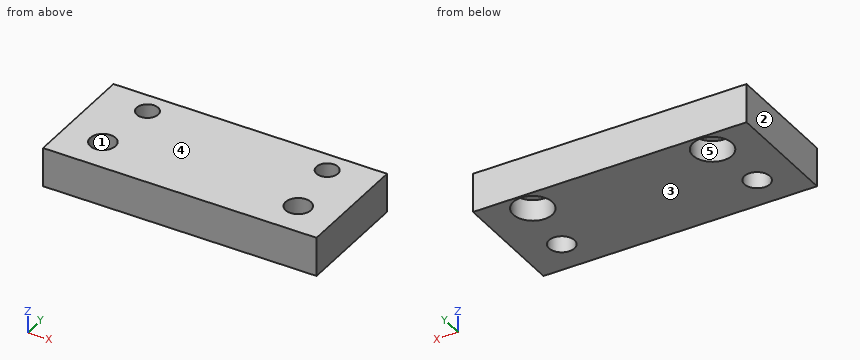
```python
from build123d import *

# Parameters (mm, degrees)
SKETCH1_W           = 70
SKETCH1_H           = 30
SKETCH1_R           = 3.25
SKETCH1_R_2         = 2.75
BOSS_EXTRUDE1_DEPTH = 10
SKETCH3_R           = 5
CUT_EXTRUDE1_DEPTH  = 5.4


with BuildPart() as part:
    # Sketch1 → Boss-Extrude1 (new body)
    with BuildSketch(Plane.XY):
        Rectangle(SKETCH1_W, SKETCH1_H)
        with Locations((-25, -6.150362319)):
            Circle(SKETCH1_R, mode=Mode.SUBTRACT)
        with Locations((25, -6.150362319)):
            Circle(SKETCH1_R, mode=Mode.SUBTRACT)
        with Locations((-23, 9.5)):
            Circle(SKETCH1_R_2, mode=Mode.SUBTRACT)
        with Locations((23, 9.5)):
            Circle(SKETCH1_R_2, mode=Mode.SUBTRACT)
    extrude(amount=BOSS_EXTRUDE1_DEPTH)

    # Sketch3 → Cut-Extrude1 (cut)
    with BuildSketch(Plane(origin=(0, 0, 0), x_dir=(-1, 0, 0), z_dir=(0, 0, -1))):
        with Locations((-23, 9.5)):
            Circle(SKETCH3_R)
        with Locations((23, 9.5)):
            Circle(SKETCH3_R)
    extrude(amount=-CUT_EXTRUDE1_DEPTH, mode=Mode.SUBTRACT)


solid = part.part
```
Verification items for the finished model (mm, model axes). Face numbers are marked on the shaded views. A direction names the side the tool comes from. Coordinates: 2 decimals unless noted, no trailing zeros. Loops run counter-clockwise (first coordinate to the right, second up) from the corner with the lowest first, then second, coordinate; pieces in that order, holes last. Notation, with made-up numbers: (-39, -13) - (-35, -13) arc R22 cw to (-35, -6) - close; hole circle Ø3 at (-34.75, 87). An arc over 180 degrees is marked (long way). Put each result on its own line as item: value.
Item 1: Draft check along X on the marked faces 1, 2 and 3. Enter one of: pulls with the +X half, pulls with the -X half, needs draft (parallel to the pull), parting line crosses it, or undercut.
Conclusion:
face 1: undercut
face 2: pulls with the -X half
face 3: needs draft
Item 2: Section check B-B (x = -25). Enter the section's corners in (y, z), then the cut area to 3 significant figures.
Conclusion:
outline: (-15, 0) - (-9.4, 0) - (-9.4, 10) - (-15, 10) - close; (-2.9, 0) - (4.92, 0) - (4.92, 5.4) - (7.61, 5.4) - (7.61, 10) - (-2.9, 10) - close; (11.39, 5.4) - (14.08, 5.4) - (14.08, 0) - (15, 0) - (15, 10) - (11.39, 10) - close
area: 168 mm2
Item 3: Set-up check for the marked faces 4 and 5: record each of +Z, -Z, +X, -X, +Y, -Y from which the full face is reachable in a straight line by a thin tool's end or side.
Conclusion:
face 4: +Z, +X, -X, +Y, -Y
face 5: -Z
Item 4: Section check C-C (z = 3). Enter the section's corners in (x, y), then the cut area to 3 significant figures.
Conclusion:
outline: (-35, -15) - (35, -15) - (35, 15) - (-35, 15) - close; hole circle Ø6.5 at (-25, -6.15); hole circle Ø10 at (-23, 9.5); hole circle Ø10 at (23, 9.5); hole circle Ø6.5 at (25, -6.15)
area: 1,880 mm2
Item 5: Section check A-A (y = 9.5). Enter the section's corners in (x, z).
Conclusion:
outline: (-35, 0) - (-28, 0) - (-28, 5.4) - (-25.75, 5.4) - (-25.75, 10) - (-35, 10) - close; (-20.25, 5.4) - (-18, 5.4) - (-18, 0) - (18, 0) - (18, 5.4) - (20.25, 5.4) - (20.25, 10) - (-20.25, 10) - close; (25.75, 5.4) - (28, 5.4) - (28, 0) - (35, 0) - (35, 10) - (25.75, 10) - close
Item 6: Gauge pin test, flat ends, axial feed: pin 1 Ø4 at (x, y) = (25, -6.15) entering from +Z; pin 2 Ø3 at (x, y) = (21.5, 10) entering from -Z. Record the tip position at first contact, or that the pin passes through.
Conclusion:
pin 1: passes through
pin 2: stops at z = 5.4
Item 7: Scan lines: line 1 along X through (y, z) = (9.5, 8.7); line 2 along X through (y, z) = (8.5, 8); line 3 along Y through (x, z) = (-23, 8). Record each from-to range of solid material in increasing order.
Conclusion:
line 1: x = -35 to -25.75, -20.25 to 20.25, 25.75 to 35
line 2: x = -35 to -25.56, -20.44 to 20.44, 25.56 to 35
line 3: y = -15 to -8.71, -3.59 to 6.75, 12.25 to 15
